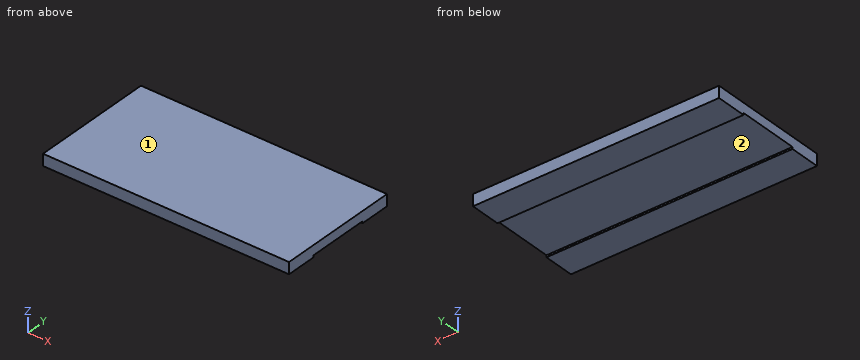
```python
from build123d import *

# Parameters (mm, degrees)
SKETCH1_W               = 203.2
SKETCH1_H               = 101.6
BOSS_EXTRUDE1_DEPTH     = 9.525
CUT_EXTRUDE1_DEPTH      = 168.059092726
CUT_EXTRUDE1_DEPTH_BACK = 228.384092726
CUT_EXTRUDE1_START      = 60.325
SKETCH2_W               = 1.5875
SKETCH2_H               = 50.8


with BuildPart() as part:
    # Sketch1 → Boss-Extrude1 (new body)
    with BuildSketch(Plane.XY):
        with Locations((101.6, 50.8)):
            Rectangle(SKETCH1_W, SKETCH1_H)
    extrude(amount=BOSS_EXTRUDE1_DEPTH)

    # Sketch2 → Cut-Extrude1 (cut, two sides: drawn at the far end of the back side and taken through both)
    with BuildSketch(Plane(origin=(0, 0, 0), x_dir=(0, 0, -1), z_dir=(1, 0, 0)).offset(CUT_EXTRUDE1_START - CUT_EXTRUDE1_DEPTH_BACK)):
        with Locations((-0.79375, 50.8)):
            Rectangle(SKETCH2_W, SKETCH2_H)
    extrude(amount=CUT_EXTRUDE1_DEPTH + CUT_EXTRUDE1_DEPTH_BACK, mode=Mode.SUBTRACT)


solid = part.part
```
For this review, take the finished solid that the model builds, in its own axes (mm). Face numbers are marked on the shaded views. Round coordinates to 2 decimals unless told otherwise and drop trailing zeros. Write each loop counter-clockwise with the first axis right and the second up, starting at its lowest first coordinate (ties: lowest second). Pieces come first, ordered by that corner, then holes. Notation, with made-up numbers: (22.5, 30.5) - (60.5, 30.5) arc R37 cw to (60.5, 68.5) - close; hole circle Ø2 at (76.5, 8). An arc over 180 degrees is marked (long way). Answer as a JSON object with one key per item and string values.
1. For pin 1 Ø12 at (x, y) = (28, 46.5) entering from -Z, flat-tipped, find the tip position at first contact; note if it passes through.
Response values:
{"pin 1": "stops at z = 1.59"}
2. We need section B-B on y = 33.5. Give the boundary of the cut face in (x, z) (1 decimal).
Response values:
{"outline": "(0, 1.6) - (203.2, 1.6) - (203.2, 9.5) - (0, 9.5) - close"}
3. We need section A-A on x = 49. Give the boundary of the cut face in (y, z) (1 decimal).
Response values:
{"outline": "(0, 0) - (25.4, 0) - (25.4, 1.6) - (76.2, 1.6) - (76.2, 0) - (101.6, 0) - (101.6, 9.5) - (0, 9.5) - close"}
4. To check wall thickness, follow line 1 along Y through (x, z) = (24.5, 1.5); line 2 along Z through (x, y) = (22.5, 54.5) (1 decimal). State the ranges of each line that lie inside material, in increasing order.
Response values:
{"line 1": "y = 0 to 25.4, 76.2 to 101.6", "line 2": "z = 1.6 to 9.5"}
5. Draft analysis for pull direction Y (two halves, no side actions). For the marked faces 1 and 2, state which applies: +Y half, -Y half, draft (parallel to the pull), parting line (faces both ways), or undercut.
Response values:
{"face 1": "draft", "face 2": "undercut"}
